from build123d import *

# Parameters (mm, degrees)
SKETCH1_W      = 50
SKETCH1_H      = 50
SKETCH1_R      = 1.5
SKETCH1_R_2    = 1.646935024
SKETCH1_R_3    = 1.908192471
SKETCH1_R_4    = 1.759080553
EXTRUDE2_DEPTH = 0.8
EXTRUDE3_DEPTH = 3
EXTRUDE4_DEPTH = 8
SKETCH4_W      = 17.5
SKETCH4_H      = 6
EXTRUDE6_DEPTH = 7
SKETCH5_W      = 17.5
SKETCH5_H      = 6
EXTRUDE7_DEPTH = 7


with BuildPart() as part:
    # Sketch1 → Extrude2 (new, symmetric)
    with BuildSketch(Plane.XY):
        Rectangle(SKETCH1_W, SKETCH1_H)
        with Locations((-22, 22)):
            Circle(SKETCH1_R, mode=Mode.SUBTRACT)
        with Locations((22, 22)):
            Circle(SKETCH1_R_2, mode=Mode.SUBTRACT)
        with Locations((22, -22)):
            Circle(SKETCH1_R_3, mode=Mode.SUBTRACT)
        with Locations((-22, -22)):
            Circle(SKETCH1_R_4, mode=Mode.SUBTRACT)
    extrude(amount=EXTRUDE2_DEPTH, both=True)

    # Sketch2 → Extrude3 (add)
    with BuildSketch(Plane.XY.offset(0.8)):
        Polygon((-20, 20), (20, -20), (-20, -20), align=None)
        Polygon((-20, 20), (20, 20), (20, -20), align=None)
    extrude(amount=EXTRUDE3_DEPTH)

    # Sketch3 → Extrude4 (add)
    with BuildSketch(Plane(origin=(0, 0, -0.8), x_dir=(-1, 0, 0), z_dir=(0, 0, -1))):
        Polygon((-20, -10), (-20, 9.2), (-12.4, 17), (-3.6, 17), (4, 9.2), (4, -10), align=None)
    extrude(amount=EXTRUDE4_DEPTH)

    # Sketch4 → Extrude6 (add)
    with BuildSketch(Plane.XY.offset(0.8)):
        with Locations((9.75, -21.5)):
            Rectangle(SKETCH4_W, SKETCH4_H)
        with Locations((-9.75, -21.5)):
            Rectangle(SKETCH4_W, SKETCH4_H)
    extrude(amount=EXTRUDE6_DEPTH)

    # Sketch5 → Extrude7 (add)
    with BuildSketch(Plane(origin=(0, 0, -0.8), x_dir=(-1, 0, 0), z_dir=(0, 0, -1))):
        with Locations((7.75, 21.5)):
            Rectangle(SKETCH5_W, SKETCH5_H)
    extrude(amount=EXTRUDE7_DEPTH)


solid = part.part
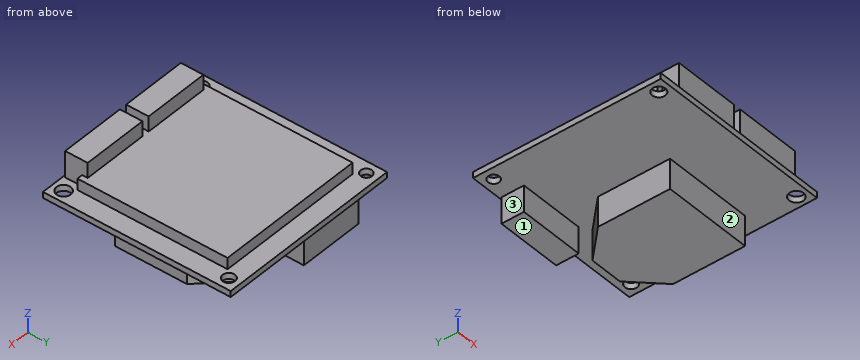
Verification items for the finished model (mm, model axes). Face numbers are marked on the shaded views. A direction names the side the tool comes from. Give positions to 0.01 mm unless a question says otherwise; leave off trailing zeros. Order: outer loops, then holes, each group sorted by start corner. A loop starts at its lowest first (then second) coordinate and runs counter-clockwise, first axis right, second up. Notation, with made-up numbers: M 49.25,8 L 84.25,8 A16 cw 84.25,37 Z; hole C 89,58.5 d3. An arc over 180 degrees is marked long. Answer as a JSON object with one key per item and string values. Group by question number.
1) Cross-section at C-C (y = -22). Enter the section's corners in (x, z).
2) Cross-section at D-D (x = -6). Enter the section's corners in (y, z).
3) Access from +Z, -Z, +X, -X, +Y, -Y to the whole of each face (thin tool, end or side, straight path). Record for the marked faces 1, 2 and 3.
4) Cross-section at B-B (x = -22). Enter the section's corners in (y, z).
5) Depth check by flat-ended pin: pin 1 Ø9 at (y, z) = (3, -6.5) entering from +X; pin 2 Ø8 at (x, z) = (-3, 2) entering from +Y; pin 3 Ø2 at (x, z) = (-11, 3) entering from -Y; pin 4 Ø6 at (x, y) = (12, 2.5) entering from +Z. Enter the tip coordinate at first touch or a pass-through.
6) Scan lines: line 1 along Y through (x, z) = (-22, 0.15); line 2 along Y through (x, z) = (22, 0.05); line 3 along Z through (x, y) = (8, -22). Record each from-to range of solid material in increasing order. Write a range as [from, to].
7) Cross-section at A-A (z = 6.75). Enter the section's corners in (x, y).
Result sheet:
{
 "1": {"outline": "M -25,-0.8 L -23.76,-0.8 L -23.76,0.8 L -25,0.8 Z; M -20.24,-0.8 L 20.09,-0.8 L 20.09,0.8 L 18.5,0.8 L 18.5,7.8 L 1,7.8 L 1,0.8 L -1,0.8 L -1,7.8 L -18.5,7.8 L -18.5,0.8 L -20.24,0.8 Z; M 23.91,-0.8 L 25,-0.8 L 25,0.8 L 23.91,0.8 Z"},
 "2": {"outline": "M -25,-0.8 L 18.5,-0.8 L 18.5,-7.8 L 24.5,-7.8 L 24.5,-0.8 L 25,-0.8 L 25,0.8 L 20,0.8 L 20,3.8 L -18.5,3.8 L -18.5,7.8 L -24.5,7.8 L -24.5,0.8 L -25,0.8 Z"},
 "3": {"face 1": "-Z, +X, -X, +Y", "face 2": "-Z, +X, -X, -Y", "face 3": "-Z, -X, +Y, -Y"},
 "4": {"outline": "M -25,-0.8 L -23.76,-0.8 L -23.76,0.8 L -25,0.8 Z; M -20.24,-0.8 L 20.5,-0.8 L 20.5,0.8 L -20.24,0.8 Z; M 23.5,-0.8 L 25,-0.8 L 25,0.8 L 23.5,0.8 Z"},
 "5": {"pin 1": "stops at x = 20", "pin 2": "stops at y = 25", "pin 3": "stops at y = -24.5", "pin 4": "stops at z = 3.8"},
 "6": {"line 1": "y = [-25, -23.76], [-20.24, 20.5], [23.5, 25]", "line 2": "y = [-25, -23.91], [-20.09, 20.35], [23.65, 25]", "line 3": "z = [-0.8, 7.8]"},
 "7": {"outline": "M -18.5,-24.5 L -1,-24.5 L -1,-18.5 L -18.5,-18.5 Z; M 1,-24.5 L 18.5,-24.5 L 18.5,-18.5 L 1,-18.5 Z"}
}
